Input: dimensioned drawing with shaded views. Units: mm. Origin: part minimum x, y, z. A direction names the side the tool comes from. Give positions to 0.01 mm unless a question says otherwise; leave off trailing zeros. Write each loop counter-clockwise with the first axis right and the second up, starting at its lowest first coordinate (ties: lowest second). Pieces come first, ordered by that corner, then holes.
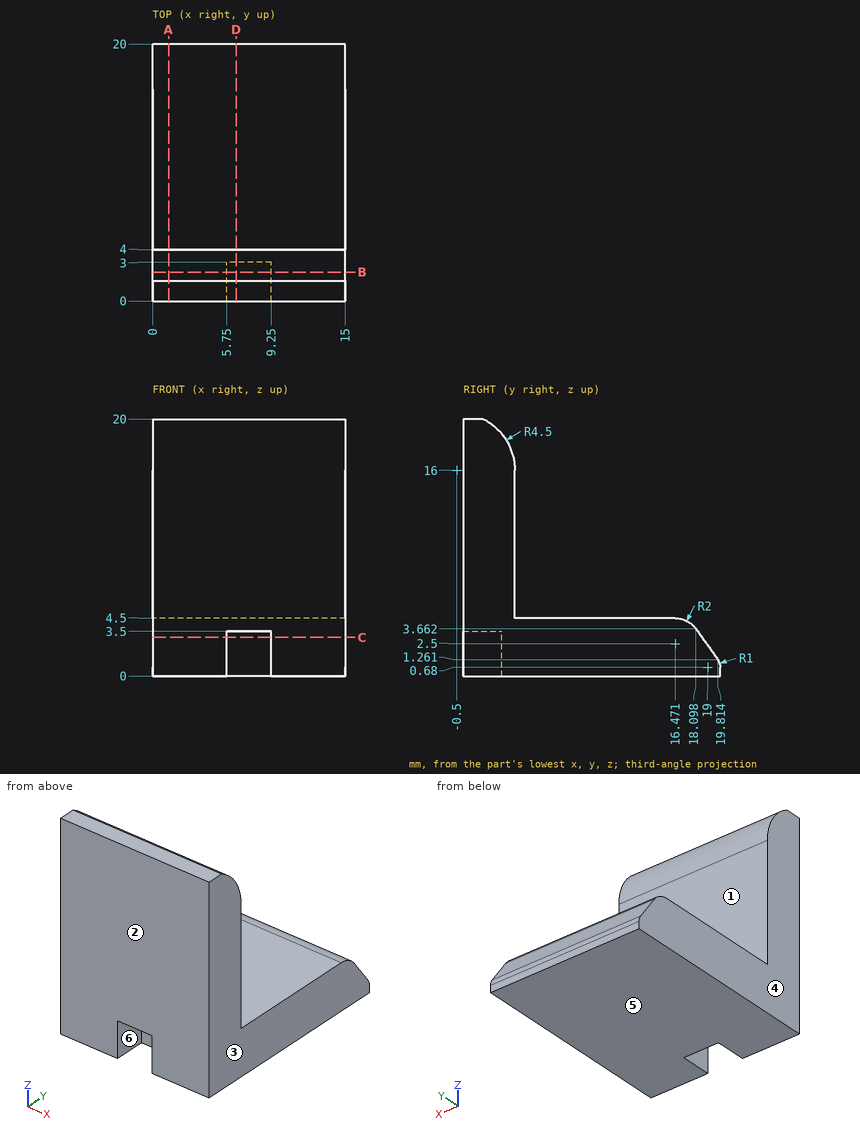
Item 1: Section D-D, the plane x = 6.5. Return the cut outline in (y, z), plus the area to 3 significant figures.
Found:
outline: (0, 3.5) - (3, 3.5) - (3, 0) - (20, 0) - (20, 0.68) arc R1 ccw to (19.81, 1.26) - (18.1, 3.66) arc R2 ccw to (16.47, 4.5) - (4, 4.5) - (4, 16) arc R4.5 ccw to (1.56, 20) - (0, 20) - close
area: 134 mm2
Item 2: Line query: L1, parallel to Z at x = 10.5, y = 16.25; L2, parallel to Y at x = 4.25, z = 16; L3, parallel to Y at x = 0.75, z = 1. Output: solid intervals per line, ascending.
Found:
L1: z = 0 to 4.5
L2: y = 0 to 4
L3: y = 0 to 19.95
Item 3: Pin query (flat end, axial travel): pin 1 Ø1 at (x, z) = (8, 1.5) entering from -Y; pin 2 Ø2 at (x, y) = (6.5, 14.5) entering from +Z; pin 3 Ø5 at (x, y) = (10.5, 6) entering from +Z; pin 4 Ø4 at (y, z) = (7.5, 12.5) entering from -X. Return the tip coordinate at first contact, or that it passes through.
Found:
pin 1: stops at y = 3
pin 2: stops at z = 4.5
pin 3: stops at z = 18.06
pin 4: passes through
Item 4: Section B-B, the plane y = 2.25. Return the cut outline in (x, z), plus the area to 3 significant figures.
Found:
outline: (0, 0) - (5.75, 0) - (5.75, 3.5) - (9.25, 3.5) - (9.25, 0) - (15, 0) - (15, 19.56) - (0, 19.56) - close
area: 281 mm2
Item 5: Section C-C, the plane z = 3. Return the cut outline in (x, y).
Found:
outline: (0, 0) - (5.75, 0) - (5.75, 3) - (9.25, 3) - (9.25, 0) - (15, 0) - (15, 18.57) - (0, 18.57) - close
Item 6: Reachability of the marked faces 1 and 2 from +Z, -Z, +X, -X, +Y, -Y: full face, straight path, thin tool, end or side. Return the list, or none.
Found:
face 1: +Z, +X, -X, +Y
face 2: +Z, -Z, +X, -X, -Y
Item 7: Section A-A, the plane x = 1.25. Return the cut outline in (y, z), plus the area to 3 significant figures.
Found:
outline: (0, 0) - (20, 0) - (20, 0.68) arc R1 ccw to (19.81, 1.26) - (18.1, 3.66) arc R2 ccw to (16.47, 4.5) - (4, 4.5) - (4, 16) arc R4.5 ccw to (1.56, 20) - (0, 20) - close
area: 145 mm2
Item 8: Pull-direction query (X, two-part tool) for the marked faces 3, 4, 5 and 6; classes: +X half, -X half, draft (parallel to the pull), parting line (faces both ways), or undercut.
Found:
face 3: +X half
face 4: -X half
face 5: draft
face 6: undercut
